from build123d import *

# Parameters (mm, degrees)
F1_DEPTH = 67.31
F3_DEPTH = 91.186
F4_R     = 145.3123956035
F5_DEPTH = 135.2049764246
F6_W     = 151.2885987759
F6_H     = 146.8262225389
F7_DEPTH = 219.4037679583
F8_R     = 29.4822475013
F9_DEPTH = 135.2059764246
F9_TAPER = -30


# Not quite as in the source:
# - a feature of the source that left no trace in its solid (it failed there, or was rolled back) is left out


with BuildPart() as f1:
    # F0 (on Top) → F1 (new body)
    with BuildSketch(Plane.XY):
        Polygon((45.1956306257, 12.500264471), (26.5868465743, 38.6269495137), (-4.4622184691, 46.6796555882), (-33.4233618988, 32.8904320264), (-46.7453428367, 3.711409783), (-38.1946583448, -27.2042223456), (-11.7722687269, -45.3906964974), (20.1584962624, -42.3383592967), (42.6568768139, -19.4754332426), align=None)
    extrude(amount=F1_DEPTH)

    # F2 (on face) → F3 (cut)
    with BuildSketch(Plane.XY.offset(67.31)):
        Polygon((13.3602926508, -6.4339778404), (13.3602926508, 6.4339778404), (3.2997197844, 14.4570169783), (-9.2456093816, 11.593627462), (-14.8288061072, 0), (-9.2456093816, -11.593627462), (3.2997197844, -14.4570169783), align=None)
    extrude(amount=-F3_DEPTH, mode=Mode.SUBTRACT)

    # F4 (on Right) → F5 (join)
    with BuildSketch(Plane.YZ):
        Circle(F4_R)
    extrude(amount=F5_DEPTH)

    # F6 (on face) → F7 (cut)
    with BuildSketch(Plane.YZ.offset(135.2049764246)):
        Rectangle(F6_W, F6_H)
    extrude(amount=-F7_DEPTH, mode=Mode.SUBTRACT)

    # F8 (on face) → F9 (cut, through all)
    with BuildSketch(Plane.YZ.offset(135.2049764246)):
        with Locations((0, 109.3934327364)):
            Circle(F8_R)
    extrude(amount=-F9_DEPTH, taper=F9_TAPER, mode=Mode.SUBTRACT)


solid = f1.part
Here's how the part is built. I have some questions about the finished solid (model axes, mm). A direction names the side the tool comes from. Round coordinates to 2 decimals unless told otherwise and drop trailing zeros. Write each loop counter-clockwise with the first axis right and the second up, starting at its lowest first coordinate (ties: lowest second). Pieces come first, ordered by that corner, then holes. Notation, with made-up numbers: (57.5, 11.5) -> (93.5, 11.5) arc R20 ccw to (93.5, 29.5) -> close; hole circle Ø4 at (19, -15). An arc over 180 degrees is marked (long way). One line per item, written item: value.
1) If I drill on line 1 (Y direction, x = 129, z = -44.5); line 2 (Y direction, x = 121, z = -67); line 3 (Z direction, x = 108.5, y = 65), over which ranges is the centre line in solid material (lowest first)? Write a range as [from, to].
Filled sheet:
line 1: y = [-138.33, -75.64], [75.64, 138.33]
line 2: y = [-128.94, -75.64], [75.64, 128.94]
line 3: z = [-129.96, -73.41], [73.41, 129.96]
2) For faces 4 (the face through (111.72, 39.76, 92.91)), 5 (the face through (69, 75.644, -1)), which set-ups out of +Z, -Z, +X, -X, +Y, -Y let a thin tool reach every point of the face, with its end or its side?
Filled sheet:
face 4: -X
face 5: +X, -X
3) We'd pull the mould along Y, two halves only. Please class faces 1 (the face through (69, -75.644, -1)), 2 (the face through (135.205, -2, -95)), 3 (the face through (66.656, -31.501, -141.857)): released by +Y, released by -Y, zero draft, split by the parting line, or undercut.
Filled sheet:
face 1: undercut
face 2: zero draft
face 3: split by the parting line
4) Suppose I cut it at A-A on z = -43. List the corners of the cut face in (x, y) for me.
Filled sheet:
outline: (0, -138.8) -> (135.2, -138.8) -> (135.2, -75.64) -> (0, -75.64) -> close; (0, 75.64) -> (135.2, 75.64) -> (135.2, 138.8) -> (0, 138.8) -> close
5) I'm going to push flat-ended pins straight in: pin 1 Ø6 at (x, y) = (52, -105) entering from +Z; pin 2 Ø4 at (x, y) = (104, -5) entering from -Z; pin 3 Ø6 at (x, z) = (50, -39.5) entering from -Y; pin 4 Ø12 at (y, z) = (-65.5, -22) entering from -X. Where does each tip first touch, or does it pass through?
Filled sheet:
pin 1: stops at z = 103.5
pin 2: stops at z = -145.28
pin 3: stops at y = -140.65
pin 4: passes through
6) Suppose I cut it at B-B on y = 0. List the corners of the cut face in (x, z) for me.
Filled sheet:
outline: (0, -145.31) -> (135.2, -145.31) -> (135.2, -73.41) -> (0, -73.41) -> close; (123.95, 73.41) -> (135.2, 73.41) -> (135.2, 79.91) -> close; (124.06, 145.31) -> (135.2, 138.88) -> (135.2, 145.31) -> close
7) Suppose I cut it at D-D on z = 0. List the corners of the cut face in (x, y) for me.
Filled sheet:
outline: (0, -145.31) -> (135.2, -145.31) -> (135.2, -75.64) -> (0, -75.64) -> close; (0, 75.64) -> (135.2, 75.64) -> (135.2, 145.31) -> (0, 145.31) -> close
8) Suppose I cut it at C-C on x = 77. List the corners of the cut face in (y, z) for me, plus the area to 3 significant figures.
Filled sheet:
outline: (-75.64, -73.41) -> (-75.64, 73.41) -> (-51.82, 73.41) arc R63.09 cw to (-58.5, 133.02) arc R145.31 ccw (long way) to (58.5, 133.02) arc R63.09 cw to (51.82, 73.41) -> (75.64, 73.41) -> (75.64, -73.41) -> close
area: 36,000 mm2
